from build123d import *

# Parameters (mm, degrees)
BOSS_EXTRUDE3_DEPTH = 15
SKETCH3_R           = 4
CUT_EXTRUDE3_DEPTH  = 14.0462
CUT_EXTRUDE4_DEPTH  = 3
CUT_EXTRUDE5_START  = -15
CUT_EXTRUDE5_DEPTH  = 12.5


with BuildPart() as part:
    # Sketch1 → Boss-Extrude3 (new body)
    with BuildSketch(Plane.YZ):
        with BuildLine():
            Line((-28.968617751, -12.789334175), (28.968617751, -12.789334175))
            ThreePointArc((28.968617751, -12.789334175), (44.579120821, 0), (35.110840206, 17.821518929))
            ThreePointArc((35.110840206, 17.821518929), (30.644623053, 21.505675602), (28.968617751, 27.047436358))
            Line((28.968617751, 27.047436358), (28.968617751, 39.053986921))
            ThreePointArc((28.968617751, 39.053986921), (26.039685563, 46.125054733), (18.968617751, 49.053986921))
            Line((18.968617751, 49.053986921), (-18.968617751, 49.053986921))
            ThreePointArc((-18.968617751, 49.053986921), (-26.039685563, 46.125054733), (-28.968617751, 39.053986921))
            Line((-28.968617751, 39.053986921), (-28.968617751, 27.047436358))
            ThreePointArc((-28.968617751, 27.047436358), (-30.644623053, 21.505675602), (-35.110840206, 17.821518929))
            ThreePointArc((-35.110840206, 17.821518929), (-44.579120821, 0), (-28.968617751, -12.789334175))
        make_face()
    extrude(amount=BOSS_EXTRUDE3_DEPTH)

    # Sketch3 → Cut-Extrude3 (cut)
    with BuildSketch(Plane.YZ.offset(15)):
        with Locations(Location((0, 3.132326373, 0), (0, 0, 270))):
            Circle(SKETCH3_R)
    extrude(amount=-CUT_EXTRUDE3_DEPTH, mode=Mode.SUBTRACT)

    # Sketch4 → Cut-Extrude4 (cut)
    with BuildSketch(Plane.YZ.offset(15)):
        with BuildLine():
            Line((-12.95, 49.053986921), (-12.95, 31.267703884))
            ThreePointArc((-12.95, 31.267703884), (0, 18.317703884), (12.95, 31.267703884))
            Line((12.95, 31.267703884), (12.95, 49.053986921))
            Line((12.95, 49.053986921), (-12.95, 49.053986921))
        make_face()
    extrude(amount=-CUT_EXTRUDE4_DEPTH, mode=Mode.SUBTRACT)

    # Sketch5 → Cut-Extrude5 (cut, symmetric)
    with BuildSketch(Plane.YZ.offset(15).offset(CUT_EXTRUDE5_START)):
        Polygon((5.466157569, 6.586954394), (-0.258716842, 9.5934717), (-5.724874411, 6.138843679), (-5.466157569, -0.322301647), (0.258716842, -3.328818953), (5.724874411, 0.125809067), align=None)
    extrude(amount=CUT_EXTRUDE5_DEPTH, both=True, mode=Mode.SUBTRACT)


solid = part.part
Input: part model. Units: mm. Frame: model coordinates. A direction names the side the tool comes from. Round coordinates to 2 decimals unless told otherwise and drop trailing zeros. Write each loop counter-clockwise with the first axis right and the second up, starting at its lowest first coordinate (ties: lowest second). Pieces come first, ordered by that corner, then holes.
1) Draft query along Z for faces 1 (the cylindrical face through (13.77, -2.43, 6.31)), 2 (the flat face through (14, -12.95, 40)), 3 (the cylindrical face through (7.395, 26.117, 46.047)). Return one class per face: pulls with the +Z half, pulls with the -Z half, needs draft (parallel to the pull), parting line crosses it, or undercut.
2) Cut plane A-A (y = 1.5). Return the cut outline in (x, z).
3) Ray query, L1, parallel to X at y = 0, z = 40.5; L2, parallel to Y at x = 3, z = 3; L3, parallel to X at y = -3.5, z = 0. Return the intervals inside material, ascending.
4) Cut plane D-D (y = -39). Return the cut outline in (x, z), then the cut area to 3 significant figures.
5) Contact query for flat-ended pins moving along their axis: P1, Ø1, axis at x = 10.5, y = -27.5, coming from the +Z side; P2, Ø3.5, axis at x = 13.5, z = 39.5, coming from the +Y side; P3, Ø8, axis at x = 5.5, z = 36, coming from the -Y side; P4, Ø6.5, axis at y = 0, z = 3.13, coming from the -X side. Output: stop coordinate, or through.
6) Reachability of faces 4 (the flat face through (7, 28.969, 33)), 5 (the flat face through (7, -28.969, 33)), 6 (the flat face through (6.338, -2.954, 7.89)), 7 (the cylindrical face through (7.395, 44.516, -0.299)), 8 (the cylindrical face through (13.52, -0.28, 18.32)) from +Z, -Z, +X, -X, +Y, -Y: full face, straight path, thin tool, end or side. Return the list, or none.
7) Cut plane C-C (z = 22). Return the cut outline in (x, y) (3 decimals).
8) Cut plane B-B (x = 10.75). Return the cut outline in (y, z).
Geometry says:
1. face 1: undercut
1. face 2: needs draft
1. face 3: pulls with the +Z half
2. outline: (0, -12.79) - (15, -12.79) - (15, -0.58) - (12.5, -0.58) - (12.5, -2.54) - (0, -2.54) - close; (0, 8.67) - (12.5, 8.67) - (12.5, 6.84) - (15, 6.84) - (15, 18.4) - (12, 18.4) - (12, 49.05) - (0, 49.05) - close
3. L1: x = 0 to 12
3. L2: y = -44.89 to -5.6, 5.61 to 44.89
3. L3: x = 12.5 to 15
4. outline: (0, -9.23) - (15, -9.23) - (15, 15.5) - (0, 15.5) - close
4. area: 371 mm2
5. P1: stops at z = 45.01
5. P2: stops at y = 28.97
5. P3: stops at y = -28.97
5. P4: passes through
6. face 4: +Z, +X, -X, +Y
6. face 5: +Z, +X, -X, -Y
6. face 6: -X
6. face 7: +X, -X, +Y
6. face 8: +Z, +X
7. outline: (0, -30.336) - (15, -30.336) - (15, -9.045) - (12, -9.045) - (12, 9.045) - (15, 9.045) - (15, 30.336) - (0, 30.336) - close
8. outline: (-35.11, 17.82) arc R15.92 ccw to (-28.97, -12.79) - (28.97, -12.79) arc R15.92 ccw to (35.11, 17.82) arc R10 cw to (28.97, 27.05) - (28.97, 39.05) arc R10 ccw to (18.97, 49.05) - (-18.97, 49.05) arc R10 ccw to (-28.97, 39.05) - (-28.97, 27.05) arc R10 cw to start; hole (-5.72, 6.14) - (-5.47, -0.32) - (0.26, -3.33) - (5.72, 0.13) - (5.47, 6.59) - (-0.26, 9.59) - close
